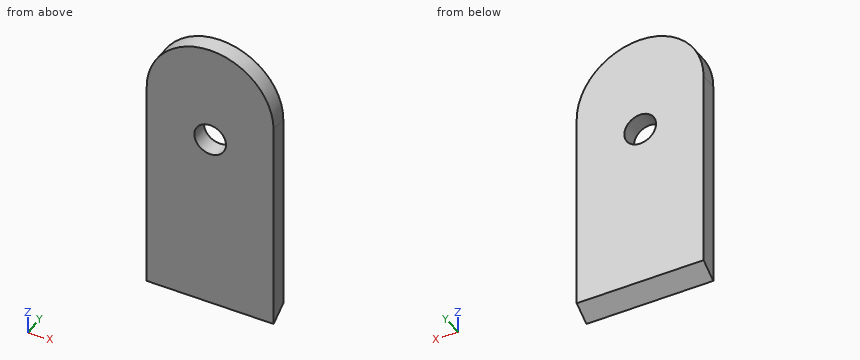
from build123d import *

# Parameters (mm, degrees)
F1_DEPTH = 19.05
F3_DEPTH = 139.701
F4_R     = 17.4625
F5_DEPTH = 19.051


with BuildPart() as f1:
    # F0 (on Front) → F1 (new body)
    with BuildSketch(Plane.XZ):
        with BuildLine():
            Line((0, 234.95), (0, 0))
            Line((0, 0), (139.7, 0))
            Line((139.7, 0), (139.7, 234.95))
            ThreePointArc((139.7, 234.95), (69.85, 304.8), (0, 234.95))
        make_face()
    extrude(amount=F1_DEPTH)

    # F2 (on face) → F3 (cut, through all)
    with BuildSketch(Plane.YZ.offset(139.7)):
        Polygon((0, 12.371215), (-19.05, 0), (0, 0), align=None)
    extrude(amount=-F3_DEPTH, mode=Mode.SUBTRACT)

    # F4 (on face) → F5 (cut, through all)
    with BuildSketch(Plane.XZ.offset(19.05)):
        with Locations((69.85, 196.85)):
            Circle(F4_R)
    extrude(amount=-F5_DEPTH, mode=Mode.SUBTRACT)


solid = f1.part
Source: CAD feature listing. Evaluate the final solid. Frame: model axes, mm. Coordinates: 2 decimals unless noted, no trailing zeros. Loops run counter-clockwise (first coordinate to the right, second up) from the corner with the lowest first, then second, coordinate; pieces in that order, holes last. Notation, with made-up numbers: (21.5, -26.75) -> (64.5, -26.75) arc R31 cw to (64.5, 2.25) -> close; hole circle Ø6 at (33, -30). An arc over 180 degrees is marked (long way). Answer in a Markdown table with one row per item. Add a question column.
Q1. Section D-D on z = 277. Return the cut outline in (x, y), and give its area (3 significant figures).
Q2. Section C-C on x = 114. Return the cut outline in (y, z).
Q3. Ray query, line 1 along X through (y, z) = (-2.5, 235.5); line 2 along X through (y, z) = (-8.75, 210); line 3 along X through (y, z) = (-7.75, 185.5). Return the intervals inside material, ascending.
Q4. Contact query for flat-ended pins moving along their axis: pin 1 Ø1 at (x, z) = (106.5, 127.5) entering from +Y; pin 2 Ø8 at (x, y) = (68, -12.5) entering from +Z; pin 3 Ø3 at (x, y) = (40, -16) entering from -Z; pin 4 Ø3 at (x, y) = (72, -5) entering from -Z. Output: stop coordinate, or through.
Q5. Section A-A on z = 196.85. Return the cut outline in (x, y), and give its area (3 significant figures).
Computed values:
| question | item | result |
|---|---|---|
| 1 | outline | (14.08, -19.05) -> (125.62, -19.05) -> (125.62, 0) -> (14.08, 0) -> close |
| 1 | area | 2,130 mm^2 |
| 2 | outline | (-19.05, 0) -> (0, 12.37) -> (0, 289.08) -> (-19.05, 289.08) -> close |
| 3 | line 1 | x = 0 to 139.7 |
| 3 | line 2 | x = 0 to 58.36, 81.34 to 139.7 |
| 3 | line 3 | x = 0 to 56.58, 83.12 to 139.7 |
| 4 | pin 1 | stops at y = 0 |
| 4 | pin 2 | stops at z = 304.8 |
| 4 | pin 3 | stops at z = 1.01 |
| 4 | pin 4 | stops at z = 8.15 |
| 5 | outline | (0, -19.05) -> (52.39, -19.05) -> (52.39, 0) -> (0, 0) -> close; (87.31, -19.05) -> (139.7, -19.05) -> (139.7, 0) -> (87.31, 0) -> close |
| 5 | area | 2,000 mm^2 |
